The model under review builds one solid part; all positions refer to its coordinate system, in mm. Give positions to 0.01 mm unless a question says otherwise; leave off trailing zeros. Order: outer loops, then holes, each group sorted by start corner. A loop starts at its lowest first (then second) coordinate and runs counter-clockwise, first axis right, second up. Notation, with made-up numbers: (77, 5) - (101, 5) arc R28 ccw to (101, 32) - close; hole circle Ø10 at (-24, 56.5). An arc over 180 degrees is marked (long way). Put each result on its own line as item: value.
```python
from build123d import *

# Parameters (mm, degrees)
F0_R     = 3.175
F1_DEPTH = 57.15
F2_DEPTH = 2.54
F3_DEPTH = 3.81
F4_DEPTH = 2.286


with BuildPart() as f1:
    # F0 (on Top) → F1 (new body)
    with BuildSketch(Plane.XY):
        Circle(F0_R)
    extrude(amount=F1_DEPTH)

    # F2 (add): a face of the model
    f2_faces = [f1.faces().sort_by_distance(p)[0] for p in [
        (0, 0, 57.15),
    ]]
    extrude(f2_faces, amount=-F2_DEPTH)

    # F3 (cut): a face of the model
    f3_faces = [f1.faces().sort_by_distance(p)[0] for p in [
        (0, 0, 57.15),
    ]]
    extrude(f3_faces, amount=-F3_DEPTH, mode=Mode.SUBTRACT)

    # F4 (cut): a face of the model
    f4_faces = [f1.faces().sort_by_distance(p)[0] for p in [
        (0, 0, 53.34),
    ]]
    extrude(f4_faces, amount=-F4_DEPTH, mode=Mode.SUBTRACT)


solid = f1.part
```
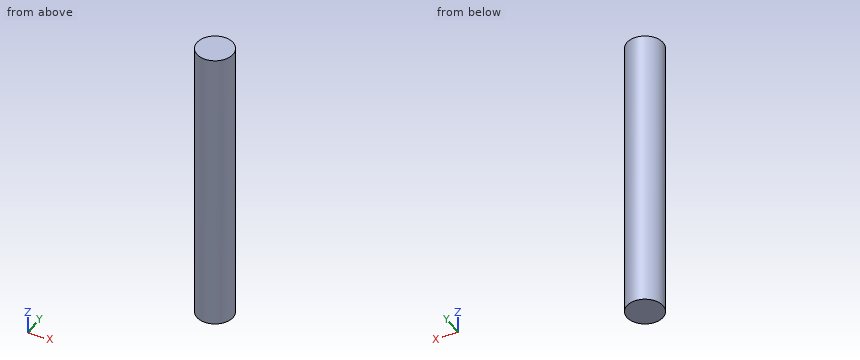
(1) Take a section at C-C, the plane y = 1.5. Write out the cut boundary in (x, z).
The answers:
outline: (-2.8, 0) - (2.8, 0) - (2.8, 51.05) - (-2.8, 51.05) - close
(2) Take a section at A-A, the plane z = 47. Write out the cut boundary in (x, y) (3 decimals), then the cut area to 3 significant figures.
The answers:
outline: circle Ø6.35 at (0, 0)
area: 31.7 mm^2
(3) Take a section at B-B, the plane x = -2.75. Write out the cut boundary in (y, z).
The answers:
outline: (-1.59, 0) - (1.59, 0) - (1.59, 51.05) - (-1.59, 51.05) - close
(4) Wall thickness on L1, parallel to Y at x = 0.25, z = 38; L2, parallel to Y at x = 1.75, z = 14; L3, parallel to X at y = 1.25, z = 18.5: over which ranges is each line inside the solid? List them lowest first.
The answers:
L1: -3.17 to 3.17
L2: -2.65 to 2.65
L3: -2.92 to 2.92
(5) Clearance check with flat-ended pins moving along their axes: pin 1 Ø2 at (y, z) = (1.5, 8) entering from -X; pin 2 Ø1.5 at (x, z) = (1.5, 29) entering from -Y. State where each tip first meets the part, or that it passes through.
The answers:
pin 1: x = -3.14
pin 2: y = -3.09
